```python
from build123d import *

# Parameters (mm, degrees)
F0_W           = 87.1929600835
F0_H           = 96.9703122973
F1_DEPTH       = 50.8
F3_D           = 6.35
F3_CBORE_D     = 12.7
F3_CBORE_DEPTH = 25.4
F5_D           = 6.35
F5_CSINK_D     = 12.7
F5_CSINK_ANGLE = 90
F6_SIZE        = 12.7


# Not quite as in the source:
# - a feature names something its author has since deleted; it is built from what else it names


with BuildPart() as f1:
    # F0 (on Front) → F1 (new body)
    with BuildSketch(Plane.XZ):
        with Locations((1.2225024402, -3.5745240748)):
            Rectangle(F0_W, F0_H)
    extrude(amount=F1_DEPTH)

    # F3 (through all)
    with Locations(Plane(origin=(0, 0, 0), x_dir=(1, 0, 0), z_dir=(0, 1, 0))):
        with Locations((0, 0)):
            CounterBoreHole(F3_D / 2, F3_CBORE_D / 2, F3_CBORE_DEPTH)

    # F5 (through all)
    with Locations(Plane(origin=(0, 0, 0), x_dir=(1, 0, 0), z_dir=(0, 1, 0))):
        with Locations((22.3049465567, -22.8805579245), (-20.5781124532, -22.8805579245), (-20.5781124532, 29.5000895858), (22.3049465567, 29.5000895858)):
            CounterSinkHole(F5_D / 2, F5_CSINK_D / 2, counter_sink_angle=F5_CSINK_ANGLE)

    # F6
    f6_edges = [f1.edges().sort_by_distance(p)[0] for p in [
        (-42.373978, -25.4, -52.05968),
        (44.818982, -25.4, -52.05968),
        (1.222502, 0, -52.05968),
        (1.222502, -50.8, -52.05968),
        (-42.373978, -25.4, 44.910632),
        (-42.373978, 0, -3.574524),
        (-42.373978, -50.8, -3.574524),
        (44.818982, -25.4, 44.910632),
        (44.818982, 0, -3.574524),
        (44.818982, -50.8, -3.574524),
        (1.222502, 0, 44.910632),
        (1.222502, -50.8, 44.910632),
    ]]
    chamfer(f6_edges, length=F6_SIZE)


solid = f1.part
```
Check sheet for the modelled part. Datum: model origin and axes. Units: mm. A direction names the side the tool comes from. Round coordinates to 2 decimals unless told otherwise and drop trailing zeros. Order: outer loops, then holes, each group sorted by start corner. A loop starts at its lowest first (then second) coordinate and runs counter-clockwise, first axis right, second up.
1) Section check C-C (y = -8). Record the boundary of the cut face in (x, z) (3 decimals), and give its area (3 significant figures).
2) Section check D-D (x = 36.5). Record the boundary of the cut face in (y, z).
3) Section check A-A (x = 0). Record the boundary of the cut face in (y, z) (3 decimals), and give its area (3 significant figures).
4) Mould release check, pull along X, two halves, no side actions. Record for faces 1 (the flat face through (38.38, -6.26, -4.08)), 2 (the cylindrical face through (-17.406, -27.321, 22.741)), 3 (the flat face through (1, -25, -52.06)): +X half, -X half, draft (parallel to the pull), parting line (faces both ways), or undercut.
5) Section check B-B (z = 0). Record the boundary of the cut face in (x, y) (3 decimals).
6) Go/stop test with flat-tipped pins: pin 1 Ø8.5 at (x, z) = (22.3, 22.88) entering from -Y; pin 2 Ø8.5 at (x, z) = (22.3, -29.5) entering from +Y; pin 3 Ø4 at (x, z) = (-20.58, 22.88) entering from +Y. Record where each tip stops, or that it passes through.
7) Tool access check on faces 4 (the flat face through (-2, -25.4, -3)), 5 (the flat face through (0.79, -6.44, -45.8)). Record the directions out of +Z, -Z, +X, -X, +Y, -Y that give a thin tool (end or side, any length) a straight path to the whole face; none if there is none.
8) Scan lines: line 1 (X direction, y = -10, z = 25); line 2 (Z direction, x = 1, y = -20); line 3 (X direction, y = -44, z = -31.5). Record each from-to range of solid material in increasing order.
Result:
1. outline: (-37.674, -39.36) - (-29.674, -47.36) - (32.119, -47.36) - (40.119, -39.36) - (40.119, 32.211) - (32.119, 40.211) - (-29.674, 40.211) - (-37.674, 32.211) - close; hole circle Ø6.35 at (-20.578, -29.5); hole circle Ø6.35 at (-20.578, 22.881); hole circle Ø12.7 at (0, 0); hole circle Ø6.35 at (22.305, -29.5); hole circle Ø6.35 at (22.305, 22.881)
1. area: 6,430 mm2
2. outline: (-46.42, -39.36) - (-38.1, -47.68) - (-12.7, -47.68) - (-4.38, -39.36) - (-4.38, 32.21) - (-12.7, 40.53) - (-38.1, 40.53) - (-46.42, 32.21) - close
3. outline: (-50.8, -39.36) - (-38.1, -52.06) - (-12.7, -52.06) - (0, -39.36) - (0, -6.35) - (-25.4, -6.35) - (-25.4, -3.175) - (-50.8, -3.175) - close; (-50.8, 3.175) - (-25.4, 3.175) - (-25.4, 6.35) - (0, 6.35) - (0, 32.211) - (-12.7, 44.911) - (-38.1, 44.911) - (-50.8, 32.211) - close
3. area: 4,120 mm2
4. face 1: +X half
4. face 2: undercut
4. face 3: draft
5. outline: (-42.374, -38.1) - (-29.674, -50.8) - (-3.175, -50.8) - (-3.175, -25.4) - (-6.35, -25.4) - (-6.35, 0) - (-29.674, 0) - (-42.374, -12.7) - close; (3.175, -50.8) - (32.119, -50.8) - (44.819, -38.1) - (44.819, -12.7) - (32.119, 0) - (6.35, 0) - (6.35, -25.4) - (3.175, -25.4) - close
6. pin 1: stops at y = -50.8
6. pin 2: stops at y = -2.1
6. pin 3: passes through
7. face 4: +Y
7. face 5: -Z, +X, -X, +Y
8. line 1: x = -39.67 to -22.94, -18.21 to 19.94, 24.67 to 42.12
8. line 2: z = -52.06 to -6.27, 6.27 to 44.91
8. line 3: x = -36.47 to -23.04, -18.11 to 19.84, 24.77 to 38.92
